Autodesk Inventor part; units mm, degrees
ref_plane "Work Plane1" through (-8, -5, 0) normal (0, 0, -1) x (0, 1, 0)
ref_plane "YZ Plane" through (0, 0, 0) normal (1, 0, 0) x (0, 1, 0)
ref_plane "XZ Plane" through (0, 0, 0) normal (0, 1, 0) x (-1, 0, 0)
sketch "Sketch1" plane through (0, 0, 0) normal (1, 0, 0) x (0, 1, 0)
  line L0 (0, 0) -> (-84.9068, 0)
  line L1 (0, -4) -> (-84.9068, -4)
  line L2 (0, -4) -> (0, -11)
  line L3 (0, -11) -> (-5, -11)
  line L4 (-5, -11) -> (-5, -7)
  line L5 (-5, -7) -> (-30, -7)
  line L6 (-30, -7) -> (-30, -4)
  dimension "d1" = 4
  dimension "d2" = 11
  dimension "d3" = 5
  dimension "d4" = 4
  dimension "d5" = 25
revolve "Revolution1" add sketch "Sketch1" angle 360 about axis through (0, 0, 0) along (0, -1, 0)
sketch "Sketch2" plane through (0, -5, 0) normal (0, -1, 0) x (1, 0, 0)
  line L0 (0, 0) -> (8, 0)
  circle A0 centre (8, 0) radius 1.5
  circle A1 centre (0, 8) radius 1.5
  circle A2 centre (-8, 0) radius 1.5
  circle A3 centre (0, -8) radius 1.5
  dimension "d7" = 8
  dimension "d8" = 3
  dimension "d11" = 360
extrude "Extrusion1" cut sketch "Sketch2" against normal blind 25.4
ref_plane "Work Plane1" through (-8, -5, 0) normal (0, 0, -1) x (0, 1, 0)
properties part number "standinNut"
Read the model definition and answer for the solid it produces. Units are mm, in the model's axes. A direction names the side the tool comes from. Coordinates: 2 decimals unless noted, no trailing zeros. Order: outer loops, then holes, each group sorted by start corner. A loop starts at its lowest first (then second) coordinate and runs counter-clockwise, first axis right, second up. Notation, with made-up numbers: (44.25, 10) - (54.25, 10) arc R24 ccw to (54.25, 42) - close; hole circle Ø5 at (58.25, 39). An arc over 180 degrees is marked (long way). Use one line per item in the form item = value.
(1) Which of the six approach directions +Z, -Z, +X, -X, +Y, -Y give full straight-line access (tool end or side, diameter ignored) to faces 1 (the face through (6.5, -2.54, 0.07)), 2 (the face through (-3.905, -15.21, 0.867))?
Computed values:
face_1 = +Y
face_2 = +Y, -Y
(2) Section C-C, the plane x = -2.25 is taken. Give the vertices of the cut face in (y, z), then the cut area to 3 significant figures.
Computed values:
outline = (-30, -6.63) - (-5, -6.63) - (-5, -10.77) - (0, -10.77) - (0, -3.31) - (-30, -3.31) - close; (-30, 3.31) - (0, 3.31) - (0, 10.77) - (-5, 10.77) - (-5, 6.63) - (-30, 6.63) - close
area = 241 mm²
(3) For a pull along Z with two mould halves and no side action, classify faces 3 (the face through (-0.325, -2.535, 6.536)), 4 (the face through (-2.681, -17.675, -6.466)), 5 (the face through (-2, -5, -7)) as pulls with the +Z half, pulls with the -Z half, needs draft (parallel to the pull), parting line crosses it, or undercut.
Computed values:
face_3 = undercut
face_4 = parting line crosses it
face_5 = needs draft
(4) Section D-D, the plane y = -14.75 is taken. Give the vertices of the cut face in (x, z).
Computed values:
outline = circle Ø14 at (0, 0); hole circle Ø8 at (0, 0)
(5) Straight lines are drawn through the part: L1, parallel to X at y = -2.8, z = 0; L2, parallel to X at y = -14, z = 0; L3, parallel to Y at x = 6.5, z = -8. For each, find the intervals that lie inside material, in ascending order.
Computed values:
L1 = -11 to -9.5, -6.5 to -4, 4 to 6.5, 9.5 to 11
L2 = -7 to -4, 4 to 7
L3 = -5 to 0
(6) Section A-A, the plane x = 0 is taken. Give the vertices of the cut face in (y, z), then the cut area to 3 significant figures.
Computed values:
outline = (-30, -7) - (-5, -7) - (-5, -6.5) - (0, -6.5) - (0, -4) - (-30, -4) - close; (-30, 4) - (0, 4) - (0, 6.5) - (-5, 6.5) - (-5, 7) - (-30, 7) - close; (-5, -11) - (0, -11) - (0, -9.5) - (-5, -9.5) - close; (-5, 9.5) - (0, 9.5) - (0, 11) - (-5, 11) - close
area = 190 mm²
(7) Section B-B, the plane z = -8 is taken. Give the vertices of the cut face in (x, y).
Computed values:
outline = (-7.55, -5) - (-1.5, -5) - (-1.5, 0) - (-7.55, 0) - close; (1.5, -5) - (7.55, -5) - (7.55, 0) - (1.5, 0) - close
(8) Given pin 1 Ø4 at (y, z) = (-8, -6) entering from -X; pin 2 Ø3 at (y, z) = (-24.5, 2) entering from -X; pin 3 Ø12 at (x, y) = (-2.5, -26.5) entering from +Z; pin 4 Ø1.8 at (x, z) = (8, 0) entering from +Y, each flat-ended and moving along its own axis, determine where each tip first touches the part or whether it passes through.
Computed values:
pin_1 = -5.74
pin_2 = -6.98
pin_3 = 7
pin_4 = through
